Could you check a few things on this drawing? It's one solid part, dimensions in mm from its lowest x, y, z. A direction names the side the tool comes from. Coordinates: 2 decimals unless noted, no trailing zeros. Write each loop counter-clockwise with the first axis right and the second up, starting at its lowest first coordinate (ties: lowest second). Pieces come first, ordered by that corner, then holes. Notation, with made-up numbers: (52.25, -3.5) - (71.25, -3.5) arc R29 ccw to (71.25, 22.5) - close; hole circle Ø9 at (14.5, -22.5). An arc over 180 degrees is marked (long way). Use one line per item in the form item = value. Start each with the question number.
(1) On a 3-axis mill with a long thin cutter (end or side, diameter ignored), from which of +Z, -Z, +X, -X, +Y, -Y can I reach the whole of each face in a straight line? I mean the marked faces 1, 2 and 3. Say none if no direction works.
(2) If we section it at D-D on z = 15.5: Please give me the cut outline in (x, y).
(3) If we section it at B-B on x = 62: Please give me the cut outline in (y, z), then the cut area to 3 significant figures.
(4) For pin 1 Ø1.5 at (x, y) = (53.5, 5) entering from +Z; pin 2 Ø6.5 at (x, z) = (62, 5) entering from +Y; pin 3 Ø3 at (y, z) = (31, 11.5) entering from +X, each with a flat end and sliding along its axis, tell me the tip position at first contact or that it passes through.
(5) If we section it at A-A on z = 5: Please give me the cut outline in (x, y), then the cut area to 3 significant figures.
(6) If I drill on probe 1 along X at (y, z) = (6, 5); probe 2 along Y at (x, z) = (42, 49.35); probe 3 along Z at (x, y) = (62, 8), over which ranges is the centre line in solid material (lowest first)? Write a range as from..to.
(7) If we section it at C-C on x = 54: Please give me the cut outline in (y, z), then the cut area to 3 significant figures.
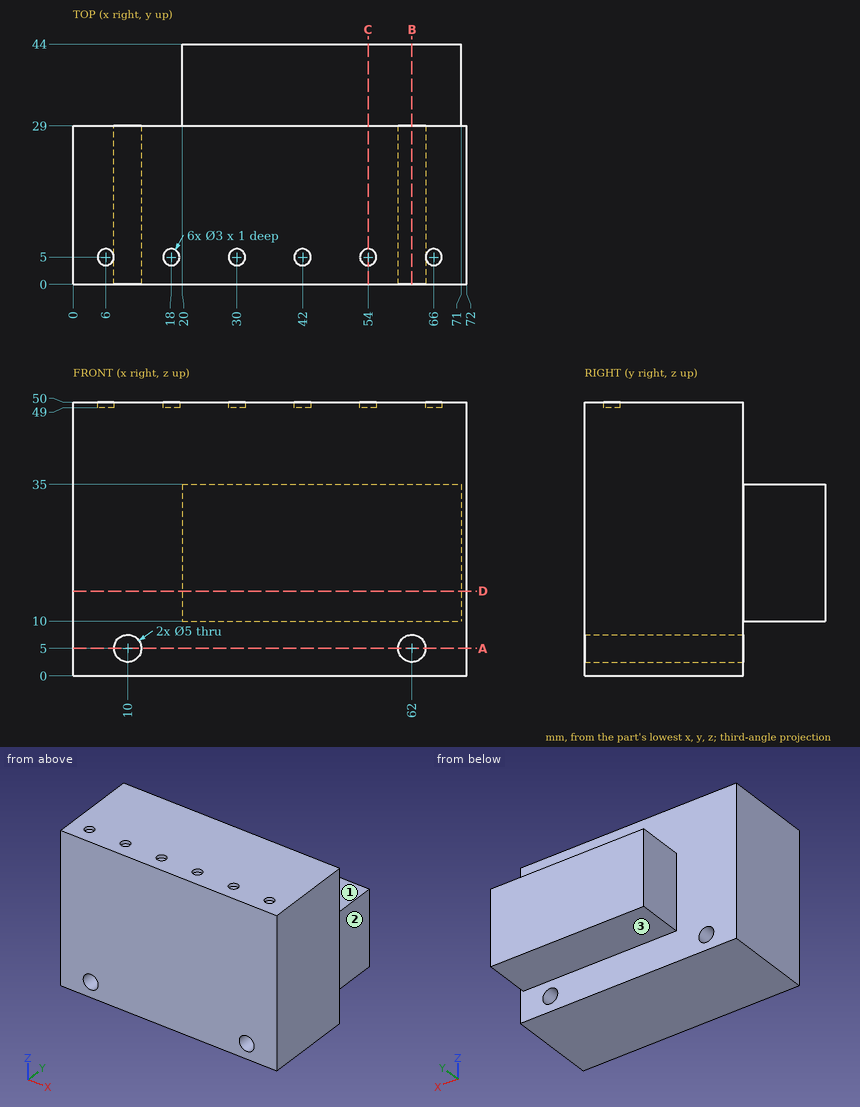
Reported:
q1.face_1 = +Z, +X, -X, +Y
q1.face_2 = +Z, -Z, +X, +Y
q1.face_3 = -Z, +X, -X, +Y
q2.outline = (0, 0) - (72, 0) - (72, 29) - (71, 29) - (71, 44) - (20, 44) - (20, 29) - (0, 29) - close
q3.outline = (0, 0) - (29, 0) - (29, 2.5) - (0, 2.5) - close; (0, 7.5) - (29, 7.5) - (29, 10) - (44, 10) - (44, 35) - (29, 35) - (29, 50) - (0, 50) - close
q3.area = 1,680 mm2
q4.pin_1 = 49
q4.pin_2 = 29
q4.pin_3 = 71
q5.outline = (0, 0) - (7.5, 0) - (7.5, 29) - (0, 29) - close; (12.5, 0) - (59.5, 0) - (59.5, 29) - (12.5, 29) - close; (64.5, 0) - (72, 0) - (72, 29) - (64.5, 29) - close
q5.area = 1,800 mm2
q6.probe_1 = 0..7.5, 12.5..59.5, 64.5..72
q6.probe_2 = 0..3.5, 6.5..29
q6.probe_3 = 0..2.5, 7.5..50
q7.outline = (0, 0) - (29, 0) - (29, 10) - (44, 10) - (44, 35) - (29, 35) - (29, 50) - (6.5, 50) - (6.5, 49) - (3.5, 49) - (3.5, 50) - (0, 50) - close
q7.area = 1,820 mm2
